```python
from build123d import *

# Parameters (mm, degrees)
SKETCH1_R             = 2.25
PLATE_THICKNESS_DEPTH = 3
EXTRUDE_2_DEPTH       = 3
SKETCH_2_3_W          = 6
SKETCH_2_3_H          = 6
SKETCH_2_3_H_2        = 2
SKETCH_2_3_W_2        = 1.95
SKETCH_2_3_H_3        = 2.000000003
SKETCH_2_3_H_4        = 1.999999997
SKETCH_2_3_H_5        = 6.000000001
CUT_EXTRUDE_1_DEPTH   = 3


with BuildPart() as part:
    # Sketch1 → Plate_thickness (new body)
    with BuildSketch(Plane.XY):
        with BuildLine():
            Line((-90, -47), (-90, -21.621))
            Line((-90, -21.621), (-43.5, -21.621))
            ThreePointArc((-43.5, -21.621), (-37.5, -15.621), (-43.5, -9.621))
            Line((-43.5, -9.621), (-90, -9.621))
            Line((-90, -9.621), (-90, 9.621))
            Line((-90, 9.621), (-43.5, 9.621))
            ThreePointArc((-43.5, 9.621), (-37.5, 15.621), (-43.5, 21.621))
            Line((-43.5, 21.621), (-90, 21.621))
            Line((-90, 21.621), (-90, 46.999999997))
            ThreePointArc((-90, 46.999999997), (-89.121320344, 49.12132034), (-87, 49.999999997))
            Line((-87, 49.999999997), (87, 49.999999997))
            ThreePointArc((87, 49.999999997), (89.121320345, 49.12132034), (90.000000002, 46.999999995))
            Line((90.000000002, 46.999999995), (90.000000002, 21.621))
            Line((90.000000002, 21.621), (43.5, 21.621))
            ThreePointArc((43.5, 21.621), (37.5, 15.621), (43.5, 9.621))
            Line((43.5, 9.621), (90, 9.621))
            Line((90, 9.621), (90, -9.621))
            Line((90, -9.621), (43.5, -9.621))
            ThreePointArc((43.5, -9.621), (37.5, -15.621), (43.5, -21.621))
            Line((43.5, -21.621), (90, -21.621))
            Line((90, -21.621), (90, -47))
            ThreePointArc((90, -47), (89.121320344, -49.121320344), (87, -50))
            Line((87, -50), (-87, -50))
            ThreePointArc((-87, -50), (-89.121320344, -49.121320344), (-90, -47))
        make_face()
        with Locations((-76, -36)):
            Circle(SKETCH1_R, mode=Mode.SUBTRACT)
        with Locations((-66, -36)):
            Circle(SKETCH1_R, mode=Mode.SUBTRACT)
        with Locations((-56, -36)):
            Circle(SKETCH1_R, mode=Mode.SUBTRACT)
        with Locations((-46, -36)):
            Circle(SKETCH1_R, mode=Mode.SUBTRACT)
        with Locations((-36, -36)):
            Circle(SKETCH1_R, mode=Mode.SUBTRACT)
        with Locations((-26, -36)):
            Circle(SKETCH1_R, mode=Mode.SUBTRACT)
        with Locations((-16, -36)):
            Circle(SKETCH1_R, mode=Mode.SUBTRACT)
        with Locations((16, -36)):
            Circle(SKETCH1_R, mode=Mode.SUBTRACT)
        with Locations((26, -36)):
            Circle(SKETCH1_R, mode=Mode.SUBTRACT)
        with Locations((36, -36)):
            Circle(SKETCH1_R, mode=Mode.SUBTRACT)
        with Locations((46, -36)):
            Circle(SKETCH1_R, mode=Mode.SUBTRACT)
        with Locations((56, -36)):
            Circle(SKETCH1_R, mode=Mode.SUBTRACT)
        with Locations((66, -36)):
            Circle(SKETCH1_R, mode=Mode.SUBTRACT)
        with Locations((76, -36)):
            Circle(SKETCH1_R, mode=Mode.SUBTRACT)
        with Locations((-76, 36)):
            Circle(SKETCH1_R, mode=Mode.SUBTRACT)
        with Locations((-66, 36)):
            Circle(SKETCH1_R, mode=Mode.SUBTRACT)
        with Locations((-56, 36)):
            Circle(SKETCH1_R, mode=Mode.SUBTRACT)
        with Locations((-46, 36)):
            Circle(SKETCH1_R, mode=Mode.SUBTRACT)
        with Locations((-36, 36)):
            Circle(SKETCH1_R, mode=Mode.SUBTRACT)
        with Locations((-26, 36)):
            Circle(SKETCH1_R, mode=Mode.SUBTRACT)
        with Locations((-16, 36)):
            Circle(SKETCH1_R, mode=Mode.SUBTRACT)
        with Locations((16, 36)):
            Circle(SKETCH1_R, mode=Mode.SUBTRACT)
        with Locations((26, 36)):
            Circle(SKETCH1_R, mode=Mode.SUBTRACT)
        with Locations((36, 36)):
            Circle(SKETCH1_R, mode=Mode.SUBTRACT)
        with Locations((46, 36)):
            Circle(SKETCH1_R, mode=Mode.SUBTRACT)
        with Locations((56, 36)):
            Circle(SKETCH1_R, mode=Mode.SUBTRACT)
        with Locations((66, 36)):
            Circle(SKETCH1_R, mode=Mode.SUBTRACT)
        with Locations((76, 36)):
            Circle(SKETCH1_R, mode=Mode.SUBTRACT)
    extrude(amount=PLATE_THICKNESS_DEPTH)

    # 草图2 → 凸台-拉伸2 (add)
    with BuildSketch(Plane.XY.offset(3)):
        Polygon((-90, 54.999999997), (-90, 46.999999997), (-48, 46.999999997), (-48, 48.999999997), (-49.95, 48.999999997), (-49.95, 54.999999997), (-60, 54.999999997), align=None)
        Polygon((-42, 48.999999997), (-42, 46.999999997), (0, 46.999999997), (42, 46.999999997), (42, 48.999999997), (40.05, 48.999999997), (40.05, 54.999999997), (30, 54.999999997), (-30, 54.999999997), (-40.05, 54.999999997), (-40.05, 48.999999997), align=None)
        Polygon((-42, 57.999999997), (-42, 54.999999997), (-40.05, 54.999999997), (-30, 54.999999997), (-30, 57.999999997), align=None)
        Polygon((-60, 57.999999997), (-60, 54.999999997), (-49.95, 54.999999997), (-48, 54.999999997), (-48, 57.999999997), align=None)
        Polygon((48, 48.999999997), (48, 46.999999997), (90, 46.999999997), (90, 54.999999997), (60, 54.999999997), (49.95, 54.999999997), (49.95, 48.999999997), align=None)
        Polygon((48, 57.999999997), (48, 54.999999997), (49.95, 54.999999997), (60, 54.999999997), (60, 57.999999997), align=None)
        Polygon((40.05, 54.999999997), (42, 54.999999997), (42, 57.999999997), (30, 57.999999997), (30, 54.999999997), align=None)
        Polygon((42, -47), (0, -47), (-42, -47), (-42, -48.999999997), (-40.05, -48.999999997), (-40.05, -54.999999997), (-30, -55), (30, -55), (40.05, -55), (40.05, -48.999999997), (42, -48.999999997), align=None)
        Polygon((90, -47), (48, -47), (48, -48.999999997), (49.95, -48.999999997), (49.95, -54.999999997), (60, -55), (90, -55), align=None)
        Polygon((-48, -48.999999997), (-48, -47), (-90, -47), (-90, -55), (-60, -55), (-49.95, -55), (-49.95, -48.999999997), align=None)
        Polygon((-48, -57.999999997), (-48, -54.999999998), (-49.95, -55), (-60, -55), (-60, -57.999999997), align=None)
        Polygon((-40.05, -55), (-42, -55), (-42, -57.999999997), (-30, -57.999999997), (-30, -54.999999997), align=None)
        Polygon((42, -57.999999997), (42, -54.999999998), (40.05, -55), (30, -55), (30, -57.999999997), align=None)
        Polygon((49.95, -55), (48, -55), (48, -57.999999997), (60, -57.999999997), (60, -54.999999997), align=None)
    extrude(amount=-EXTRUDE_2_DEPTH)

    # 草图2<3> → 切除-拉伸1 (cut)
    with BuildSketch(Plane.XY.offset(3)):
        with Locations((-45, 51.999999997)):
            Rectangle(SKETCH_2_3_W, SKETCH_2_3_H)
        with Locations((-45, 47.999999997)):
            Rectangle(SKETCH_2_3_W, SKETCH_2_3_H_2)
        with Locations((-45, 45.999999997)):
            Rectangle(SKETCH_2_3_W, SKETCH_2_3_H_2)
        with Locations((-41.025, 51.999999997)):
            Rectangle(SKETCH_2_3_W_2, SKETCH_2_3_H)
        with Locations((-48.975, 51.999999997)):
            Rectangle(SKETCH_2_3_W_2, SKETCH_2_3_H)
        with Locations((41.025, 51.999999997)):
            Rectangle(SKETCH_2_3_W_2, SKETCH_2_3_H)
        with Locations((45, 51.999999997)):
            Rectangle(SKETCH_2_3_W, SKETCH_2_3_H)
        with Locations((48.975, 51.999999997)):
            Rectangle(SKETCH_2_3_W_2, SKETCH_2_3_H)
        with Locations((45, 47.999999997)):
            Rectangle(SKETCH_2_3_W, SKETCH_2_3_H_2)
        with Locations((45, 45.999999997)):
            Rectangle(SKETCH_2_3_W, SKETCH_2_3_H_2)
        with Locations((45, -45.999999999)):
            Rectangle(SKETCH_2_3_W, SKETCH_2_3_H_3)
        with Locations((45, -47.999999999)):
            Rectangle(SKETCH_2_3_W, SKETCH_2_3_H_4)
        Polygon((48, -48.999999997), (42, -48.999999997), (42, -54.999999998), (48, -55), align=None)
        Polygon((42, -54.999999998), (42, -48.999999997), (40.05, -48.999999997), (40.05, -54.999999997), align=None)
        Polygon((49.95, -48.999999997), (48, -48.999999997), (48, -54.999999998), (49.95, -55), align=None)
        with Locations((-45, -45.999999999)):
            Rectangle(SKETCH_2_3_W, SKETCH_2_3_H_3)
        with Locations((-45, -47.999999999)):
            Rectangle(SKETCH_2_3_W, SKETCH_2_3_H_4)
        with Locations((-45, -51.999999998)):
            Rectangle(SKETCH_2_3_W, SKETCH_2_3_H_5)
        Polygon((-48, -54.999999998), (-48, -48.999999997), (-49.95, -48.999999997), (-49.95, -54.999999997), align=None)
        Polygon((-40.05, -48.999999997), (-42, -48.999999997), (-42, -54.999999998), (-40.05, -55), align=None)
        with BuildLine():
            ThreePointArc((-10.16, 7.39), (-9.099339828, 7.829339828), (-8.66, 8.89))
            Line((-8.66, 8.89), (-10.16, 8.89))
            Line((-10.16, 8.89), (-10.16, 7.39))
        make_face()
        with BuildLine():
            Line((-10.16, 8.89), (-8.66, 8.89))
            ThreePointArc((-8.66, 8.89), (-11.220660172, 9.950660172), (-10.16, 7.39))
            Line((-10.16, 7.39), (-10.16, 8.89))
        make_face()
        with BuildLine():
            ThreePointArc((11.66, 8.89), (10.16, 10.39), (8.66, 8.89))
            Line((8.66, 8.89), (10.16, 8.89))
            Line((10.16, 8.89), (10.16, 7.39))
            ThreePointArc((10.16, 7.39), (11.220660172, 7.829339828), (11.66, 8.89))
        make_face()
        with BuildLine():
            Line((10.16, 8.89), (8.66, 8.89))
            ThreePointArc((8.66, 8.89), (9.099339828, 7.829339828), (10.16, 7.39))
            Line((10.16, 7.39), (10.16, 8.89))
        make_face()
        with BuildLine():
            ThreePointArc((10.16, -7.39), (9.099339828, -7.829339828), (8.66, -8.89))
            Line((8.66, -8.89), (10.16, -8.89))
            Line((10.16, -8.89), (10.16, -7.39))
        make_face()
        with BuildLine():
            Line((10.16, -8.89), (8.66, -8.89))
            ThreePointArc((8.66, -8.89), (10.16, -10.39), (11.66, -8.89))
            ThreePointArc((11.66, -8.89), (11.220660172, -7.829339828), (10.16, -7.39))
            Line((10.16, -7.39), (10.16, -8.89))
        make_face()
        with BuildLine():
            ThreePointArc((-10.16, -7.39), (-11.220660172, -9.950660172), (-8.66, -8.89))
            Line((-8.66, -8.89), (-10.16, -8.89))
            Line((-10.16, -8.89), (-10.16, -7.39))
        make_face()
        with BuildLine():
            Line((-10.16, -8.89), (-8.66, -8.89))
            ThreePointArc((-8.66, -8.89), (-9.099339828, -7.829339828), (-10.16, -7.39))
            Line((-10.16, -7.39), (-10.16, -8.89))
        make_face()
    extrude(amount=-CUT_EXTRUDE_1_DEPTH, mode=Mode.SUBTRACT)


solid = part.part
```
Can you work these out from the model? Positions are in its coordinate system, mm. Round coordinates to 2 decimals unless told otherwise and drop trailing zeros. Loops run counter-clockwise (first coordinate to the right, second up) from the corner with the lowest first, then second, coordinate; pieces in that order, holes last. Notation, with made-up numbers: M 57.5,68 L 107.5,68 A30 ccw 107.5,94 Z; hole C 0.5,8 d3. An arc over 180 degrees is marked long. Answer as a JSON object with one key per item and string values. Group by question number.
Q1. We'd pull the mould along X, two halves only. Please class faces 1 (the flat face through (-1, 1, 3)), 2 (the cylindrical face through (37.5, 15.75, 1.48)), 3 (the cylindrical face through (-37.5, -15.75, 1.48)), 4 (the cylindrical face through (17.21, -34.103, 1.479)): +X half, -X half, draft (parallel to the pull), parting line (faces both ways), or undercut.
Q2. Imagine slicing it at C-C, the plane z = 0.95. Count the separate pieces of the cut face and the enclosed holes in it, then the cut area to 3 significant figures.
Q3. Please list where these lines run through material, in increasing order: L1, parallel to X at y = 52.5, z = 0.2; L2, parallel to Y at x = 69, z = 0.4; L3, parallel to Y at x = 56, z = 1.15.
Q4. Imagine slicing it at B-B, the plane x = 46. Please give me the cut outline in (y, z), then the cut area to 3 significant figures.
Q5. Imagine slicing it at A-A, the plane x = -26. Please give me the cut outline in (y, z), then the cut area to 3 significant figures.
Q6. Will these pins go through, and if not, where does the flat tip stop? pin 1 (1.5 mm diameter, centred on x = -44, z = 2, fed in from +Y); pin 2 (1.5 mm diameter, centred on x = -70.5, z = 2, fed in from +Y); pin 3 (1.5 mm diameter, centred on x = -68.5, z = 2, fed in from -Y).
Findings:
{
 "1": {"face 1": "draft", "face 2": "+X half", "face 3": "-X half", "face 4": "undercut"},
 "2": {"separate pieces": "1", "enclosed holes": "32", "area": "16,800 mm2"},
 "3": {"L1": "x = -90 to -49.95, -40.05 to 40.05, 49.95 to 90", "L2": "y = -55 to -21.62, -9.62 to 9.62, 21.62 to 55", "L3": "y = -58 to -38.25, -33.75 to -21.62, -9.62 to 9.62, 21.62 to 33.75, 38.25 to 58"},
 "4": {"outline": "M -45,0 L -38.25,0 L -38.25,3 L -45,3 Z; M -33.75,0 L -21.62,0 L -21.62,3 L -33.75,3 Z; M -9.62,0 L 9.62,0 L 9.62,3 L -9.62,3 Z; M 21.62,0 L 33.75,0 L 33.75,3 L 21.62,3 Z; M 38.25,0 L 45,0 L 45,3 L 38.25,3 Z", "area": "171 mm2"},
 "5": {"outline": "M -55,0 L -38.25,0 L -38.25,3 L -55,3 Z; M -33.75,0 L 33.75,0 L 33.75,3 L -33.75,3 Z; M 38.25,0 L 55,0 L 55,3 L 38.25,3 Z", "area": "303 mm2"},
 "6": {"pin 1": "stops at y = 45", "pin 2": "stops at y = 55", "pin 3": "stops at y = -55"}
}
